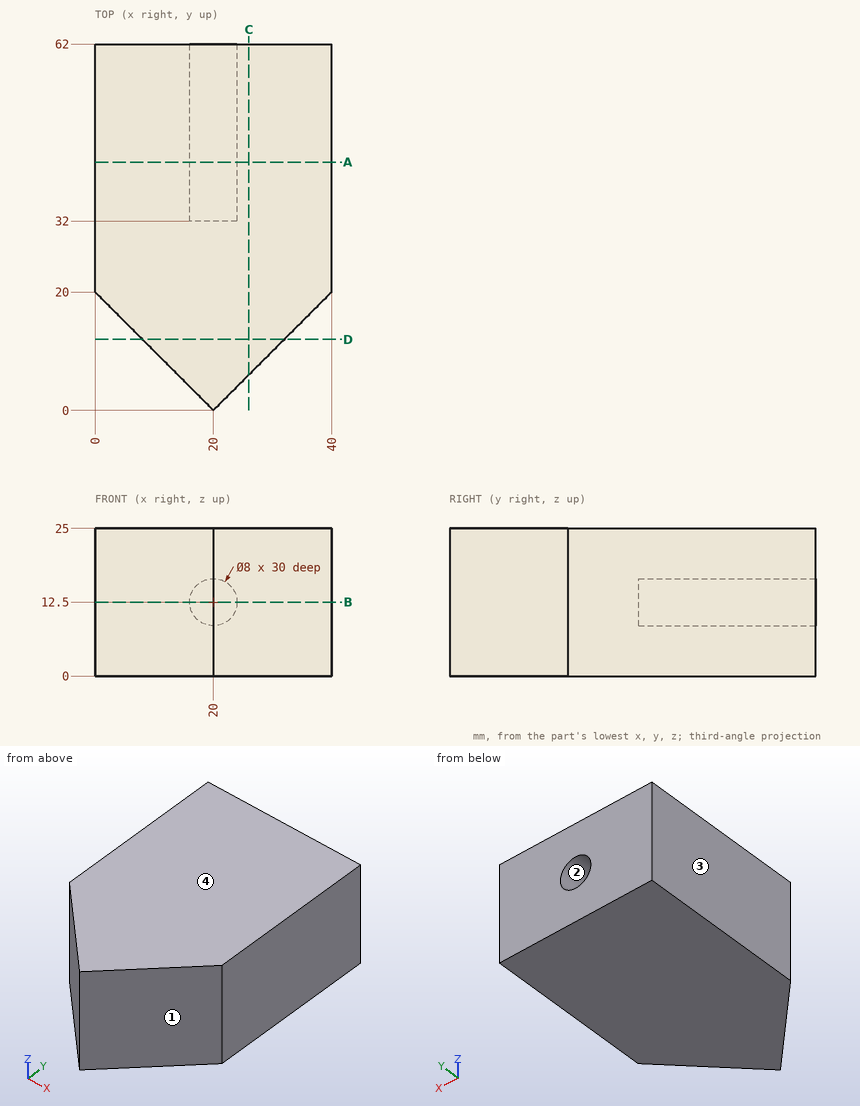
The figure shows three views and two pictorial views of one solid part (mm, origin at its lowest corner). Answer the questions. Give positions to 0.01 mm unless a question says otherwise; leave off trailing zeros. Write each loop counter-clockwise with the first axis right and the second up, starting at its lowest first coordinate (ties: lowest second). Pieces come first, ordered by that corner, then holes. Notation, with made-up numbers: (-22, 86) - (33, 86) arc R26 ccw to (33, 112) - close; hole circle Ø10 at (64, 81.25). An arc over 180 degrees is marked (long way). Use one line per item in the form item = value.
1. A cutting plane is placed at B-B (z = 12.5). Write down the section's boundary in (x, y).
Filled in:
outline = (0, 20) - (20, 0) - (40, 20) - (40, 62) - (24, 62) - (24, 32) - (16, 32) - (16, 62) - (0, 62) - close
2. A cutting plane is placed at A-A (y = 42). Write down the section's boundary in (x, z), and give its area (3 significant figures).
Filled in:
outline = (0, 0) - (40, 0) - (40, 25) - (0, 25) - close; hole circle Ø8 at (20, 12.5)
area = 950 mm^2
3. Each of these flat-tipped pins is pushed along its axis until it touches: pin 1 Ø2 at (x, z) = (13, 17) entering from -Y; pin 2 Ø12 at (x, y) = (36, 12) entering from -Z; pin 3 Ø4 at (x, z) = (25, 6) entering from -Y; pin 4 Ø2.5 at (x, z) = (19.5, 14.5) entering from +Y. Where does it stop, or does it pass through?
Filled in:
pin_1 = 6
pin_2 = 0
pin_3 = 3
pin_4 = 32
4. Determine the mould class of the marked faces 1, 2, 3 and 4 for opening direction X: released by +X, released by -X, zero draft, split by the parting line, or undercut.
Filled in:
face_1 = released by +X
face_2 = undercut
face_3 = released by -X
face_4 = zero draft
5. A cutting plane is placed at C-C (x = 26). Write down the section's boundary in (y, z), and give its area (3 significant figures).
Filled in:
outline = (6, 0) - (62, 0) - (62, 25) - (6, 25) - close
area = 1,400 mm^2
6. A cutting plane is placed at D-D (y = 12). Write down the section's boundary in (x, z), and give its area (3 significant figures).
Filled in:
outline = (8, 0) - (32, 0) - (32, 25) - (8, 25) - close
area = 600 mm^2
7. Consider L1, parallel to X at y = 40, z = 12.5; L2, parallel to Z at x = 20, y = 51; L3, parallel to Y at x = 4, z = 8.25. Determine where each line is inside the solid, lowest interval first.
Filled in:
L1 = 0 to 16, 24 to 40
L2 = 0 to 8.5, 16.5 to 25
L3 = 16 to 62
